Build history of the part. All positions in model axes, mm. Round coordinates to 2 decimals unless told otherwise and drop trailing zeros. Write each loop counter-clockwise with the first axis right and the second up, starting at its lowest first coordinate (ties: lowest second). Pieces come first, ordered by that corner, then holes.
from build123d import *

# Parameters (mm, degrees)
BOSS_EXTRUDE1_DEPTH     = 2.54
SKETCH2_R               = 5
CUT_EXTRUDE1_DEPTH      = 1
CUT_EXTRUDE1_DEPTH_BACK = 3.54


with BuildPart() as part:
    # Sketch1 → Boss-Extrude1 (new body)
    with BuildSketch(Plane(origin=(0, 0, 0), x_dir=(1, 0, 0), z_dir=(0, 1, 0))):
        with BuildLine():
            Line((-89.636017598, 11), (-11.963982402, 11))
            ThreePointArc((-11.963982402, 11), (0, 16.252288298), (11.963982402, 11))
            Line((11.963982402, 11), (89.636017598, 11))
            ThreePointArc((89.636017598, 11), (117.852288298, 0), (89.636017598, -11))
            Line((89.636017598, -11), (11.963982402, -11))
            ThreePointArc((11.963982402, -11), (0, -16.252288298), (-11.963982402, -11))
            Line((-11.963982402, -11), (-89.636017598, -11))
            ThreePointArc((-89.636017598, -11), (-117.852288298, 0), (-89.636017598, 11))
        make_face()
    extrude(amount=BOSS_EXTRUDE1_DEPTH)

    # Sketch2 → Cut-Extrude1 (cut, two sides)
    with BuildSketch(Plane(origin=(0, 2.54, 0), x_dir=(1, 0, 0), z_dir=(0, 1, 0))) as cut_extrude1_sk:
        with Locations((-101.6, 0)):
            Circle(SKETCH2_R)
        with Locations((101.6, 0)):
            Circle(SKETCH2_R)
        Circle(SKETCH2_R)
    extrude(amount=CUT_EXTRUDE1_DEPTH, mode=Mode.SUBTRACT)
    extrude(cut_extrude1_sk.sketch, amount=-CUT_EXTRUDE1_DEPTH_BACK, mode=Mode.SUBTRACT)


solid = part.part
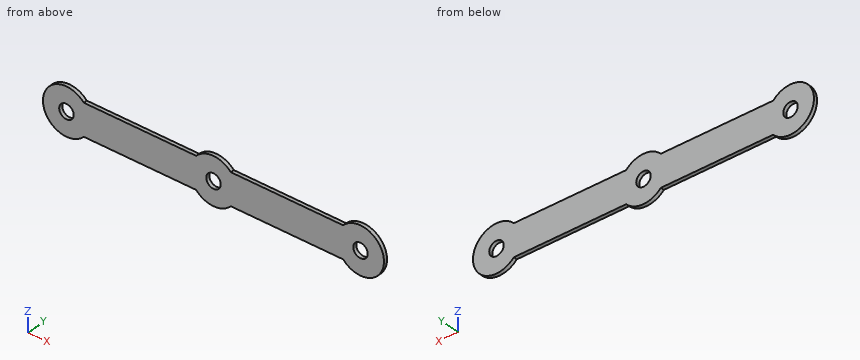
1) Wall check: L1, parallel to X at y = 1, z = -0.5; L2, parallel to Z at x = 101.6, y = 0.6; L3, parallel to X at y = 0.5, z = -4. Give the ranges that are in metal, low to high.
Results:
L1: x = -117.84 to -106.57, -96.63 to -4.97, 4.97 to 96.63, 106.57 to 117.84
L2: z = -16.25 to -5, 5 to 16.25
L3: x = -117.35 to -104.6, -98.6 to -3, 3 to 98.6, 104.6 to 117.35
2) Slice it at B-B (x = -101.6). Write the cut outline in (y, z).
Results:
outline: (0, -16.25) - (2.54, -16.25) - (2.54, -5) - (0, -5) - close; (0, 5) - (2.54, 5) - (2.54, 16.25) - (0, 16.25) - close
3) Slice it at D-D (x = 17). Write the cut outline in (y, z), plus the area to 3 significant figures.
Results:
outline: (0, -11) - (2.54, -11) - (2.54, 11) - (0, 11) - close
area: 55.9 mm2
4) Pin check, flat tips, straight feed: pin 1 Ø0.8 at (x, y) = (55.5, 1.5) entering from -Z; pin 2 Ø6 at (x, z) = (101.6, 0) entering from +Y; pin 3 Ø0.8 at (x, y) = (46.5, 1) entering from +Z. Stop position of each tip, or through.
Results:
pin 1: stops at z = -11
pin 2: passes through
pin 3: stops at z = 11
5) Slice it at C-C (y = 2.15). Write the cut outline in (x, z).
Results:
outline: (-89.64, -11) - (-11.96, -11) arc R16.25 ccw to (11.96, -11) - (89.64, -11) arc R16.25 ccw (long way) to (89.64, 11) - (11.96, 11) arc R16.25 ccw to (-11.96, 11) - (-89.64, 11) arc R16.25 ccw (long way) to start; hole circle Ø10 at (-101.6, 0); hole circle Ø10 at (0, 0); hole circle Ø10 at (101.6, 0)
6) Slice it at A-A (z = 0). Write the cut outline in (x, y), plus the area to 3 significant figures.
Results:
outline: (-117.85, 0) - (-106.6, 0) - (-106.6, 2.54) - (-117.85, 2.54) - close; (-96.6, 0) - (-5, 0) - (-5, 2.54) - (-96.6, 2.54) - close; (5, 0) - (96.6, 0) - (96.6, 2.54) - (5, 2.54) - close; (106.6, 0) - (117.85, 0) - (117.85, 2.54) - (106.6, 2.54) - close
area: 522 mm2
